from build123d import *

# Parameters (mm, degrees)
BOSS_EXTRUDE1_DEPTH = 50
CUT_EXTRUDE9_START  = -2
SKETCH3_W           = 96
SKETCH3_H           = 45
CUT_EXTRUDE9_DEPTH  = 121.474487139
SKETCH4_R           = 2.5
CUT_EXTRUDE10_DEPTH = 122.509301877


with BuildPart() as part:
    # Sketch1 → Boss-Extrude1 (new body)
    with BuildSketch(Plane.XY):
        Polygon((0, 0.250965251), (0, 7.586872587), (100, 47.586872587), (100, -2.413127413), (0, -2.413127413), align=None)
    extrude(amount=BOSS_EXTRUDE1_DEPTH)

    # Sketch3 → Cut-Extrude9 (cut, through all)
    with BuildSketch(Plane.XZ.offset(2.413127413).offset(CUT_EXTRUDE9_START)):
        with Locations((50, 25)):
            Rectangle(SKETCH3_W, SKETCH3_H)
    extrude(amount=-CUT_EXTRUDE9_DEPTH, mode=Mode.SUBTRACT)

    # Sketch4 → Cut-Extrude10 (cut, through all)
    with BuildSketch(Plane(origin=(0, 0, 0), x_dir=(-1, 0, 0), z_dir=(0, 0, -1))):
        with Locations((-5.962912018, 3.549784605)):
            Circle(SKETCH4_R)
    extrude(amount=-CUT_EXTRUDE10_DEPTH, mode=Mode.SUBTRACT)


solid = part.part
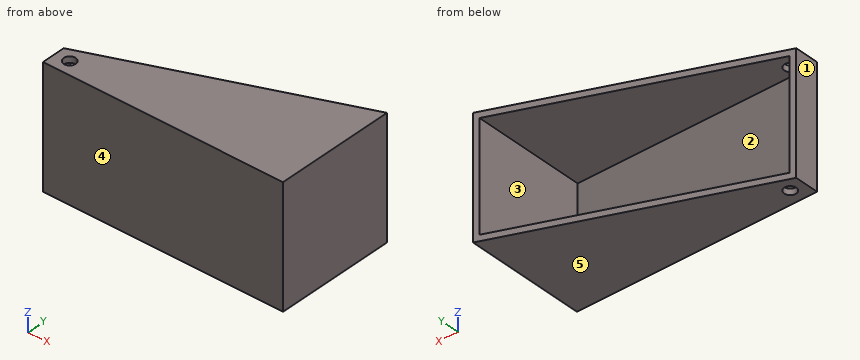
Work out the finished part from the listing and answer in its coordinate system (mm). Face numbers are marked on the shaded views. A direction names the side the tool comes from. Give positions to 0.01 mm unless a question says otherwise; leave off trailing zeros. Loops run counter-clockwise (first coordinate to the right, second up) from the corner with the lowest first, then second, coordinate; pieces in that order, holes last. Notation, with made-up numbers: (78.25, 60) - (91.25, 60) arc R25 ccw to (91.25, 94) - close; hole circle Ø1 at (8.25, 41.25). An arc over 180 degrees is marked (long way). Answer in a Markdown table with one row per item.
(1) Consider L1, parallel to Z at x = 78.5, y = 31; L2, parallel to X at y = 6, z = 45.5; L3, parallel to X at y = 23, z = 26. Determine where each line is inside the solid, lowest interval first. Write a range as [from, to].
Results list:
| item | result |
|---|---|
| L1 | z = [0, 2.5], [47.5, 50] |
| L2 | x = [0, 2], [98, 100] |
| L3 | x = [98, 100] |
(2) Section A-A (z = 19) is taken. Give the vertices of the cut face in (x, y).
Results list:
| item | result |
|---|---|
| outline | (0, -2.41) - (100, -2.41) - (100, 47.59) - (98, 46.79) - (98, -0.41) - (2, -0.41) - (2, 8.39) - (0, 7.59) - close |
(3) A tool of negligible diameter and unlimited length cuts with its end or side. For the marked faces 1 and 2, from which of +Z, -Z, +X, -X, +Y, -Y can it reach the whole face along a straight path? Write none if from no direction.
Results list:
| item | result |
|---|---|
| face 1 | +Z, -Z, -X, +Y, -Y |
| face 2 | +Y |
(4) For a pull along Z with two mould halves and no side action, classify the marked faces 3, 4 and 5 as pulls with the +Z half, pulls with the -Z half, needs draft (parallel to the pull), parting line crosses it, or undercut.
Results list:
| item | result |
|---|---|
| face 3 | undercut |
| face 4 | needs draft |
| face 5 | pulls with the -Z half |
(5) Section B-B (x = 34) is taken. Give the vertices of the cut face in (y, z), and give its area (3 significant figures).
Results list:
| item | result |
|---|---|
| outline | (-2.41, 0) - (21.19, 0) - (21.19, 2.5) - (-0.41, 2.5) - (-0.41, 47.5) - (21.19, 47.5) - (21.19, 50) - (-2.41, 50) - close |
| area | 208 mm² |
(6) Flat-ended cylindrical pins translate along their axes: pin 1 Ø6.5 at (x, y) = (5.96, 3.55) entering from +Z; pin 2 Ø3 at (y, z) = (18.5, 38.5) entering from -X; pin 3 Ø13.5 at (x, z) = (42.5, 27) entering from +Y; pin 4 Ø10 at (x, z) = (36, 43) entering from +Y. Find the tip coordinate at first contact, or state that the pin passes through.
Results list:
| item | result |
|---|---|
| pin 1 | stops at z = 50 |
| pin 2 | stops at x = 98 |
| pin 3 | stops at y = -0.41 |
| pin 4 | stops at y = 22.86 |
